Autodesk Inventor part; units mm, degrees
ref_plane "YZ Plane" through (0, 0, 0) normal (1, 0, 0) x (0, 1, 0)
ref_plane "XZ Plane" through (0, 0, 0) normal (0, 1, 0) x (-1, 0, 0)
ref_plane "XY Plane" through (0, 0, 0) normal (0, 0, 1) x (1, 0, 0)
sketch "スケッチ1" plane through (0, 0, 0) normal (0, 0, 1) x (1, 0, 0)
  circle A0 centre (89.1334, 60.2981) radius 8.025
  arc A1 (110.4927, 37.2495) -> (107.5312, 48.5254) centre (107.6371, 42.5263) ccw
  arc A2 (106.5859, 49.1517) -> (107.5312, 48.5254) centre (107.5135, 49.5253) ccw
  line L0 (106.5859, 49.1517) -> (100.2878, 64.7903)
  arc A3 (100.2878, 64.7903) -> (96.6592, 69.6769) centre (89.1334, 60.2981) ccw
  line L1 (96.6592, 69.6769) -> (61.7006, 97.7286)
  arc A4 (61.7006, 97.7286) -> (50.6268, 86.1987) centre (56.6782, 91.4695) ccw
  line L2 (50.6268, 86.1987) -> (79.2604, 53.3248)
  arc A5 (79.3697, 53.1725) -> (79.2604, 53.3248) centre (78.5063, 52.668) ccw
  line L3 (79.3697, 53.1725) -> (86.5144, 40.9457)
  arc A6 (86.5144, 40.9457) -> (87.5386, 39.6454) centre (91.6947, 43.9728) ccw
  line L4 (87.5386, 39.6454) -> (105.5692, 22.328)
  arc A7 (105.5692, 22.328) -> (111.1188, 32.4913) centre (109.7254, 26.6553) ccw
  arc A8 (110.3596, 33.3335) -> (111.1188, 32.4913) centre (111.3511, 33.464) ccw
  line L5 (110.3596, 33.3335) -> (109.9772, 36.2396)
  arc A9 (110.4927, 37.2495) -> (109.9772, 36.2396) centre (110.9687, 36.37) ccw
  circle A10 centre (68.955, 78.0364) radius 1.25
  circle A11 centre (109.7254, 26.6553) radius 3.025
  circle A12 centre (107.6371, 42.5263) radius 3.025
  circle A13 centre (91.6947, 43.9728) radius 3.025
  circle A14 centre (56.6782, 91.4695) radius 1.25
  arc A15 (83.1457, 72.8964) -> (83.5589, 72.581) centre (90.3437, 81.8972) ccw
  arc A16 (83.1457, 72.8964) -> (74.4673, 77.9243) centre (62.1124, 46.5952) ccw
  arc A17 (74.4673, 77.9243) -> (73.1203, 77.1926) centre (74.1004, 76.994) ccw
  arc A18 (68.4822, 73.8128) -> (73.1203, 77.1926) centre (68.955, 78.0364) ccw
  arc A19 (68.4822, 73.8128) -> (67.371, 72.8351) centre (68.3709, 72.819) ccw
  line L6 (67.371, 72.8351) -> (67.3568, 71.9495)
  arc A20 (67.3568, 71.9495) -> (67.6026, 71.2766) centre (68.3567, 71.9334) ccw
  line L7 (67.6026, 71.2766) -> (75.5898, 62.1066)
  arc A21 (75.5898, 62.1066) -> (77.3258, 62.5741) centre (76.3438, 62.7634) ccw
  arc A22 (83.4434, 70.8917) -> (77.3258, 62.5741) centre (89.1334, 60.2981) ccw
  arc A23 (83.4434, 70.8917) -> (83.5589, 72.581) centre (82.9702, 71.7727) ccw
  arc A24 (97.4697, 45.6005) -> (95.5411, 48.5777) centre (91.6947, 43.9728) ccw
  arc A25 (97.4697, 45.6005) -> (98.3419, 44.8759) centre (98.4322, 45.8718) ccw
  line L8 (98.3419, 44.8759) -> (101.261, 44.611)
  arc A26 (101.261, 44.611) -> (102.2493, 45.1668) centre (101.3514, 45.6069) ccw
  arc A27 (103.6511, 47.011) -> (102.2493, 45.1668) centre (107.6371, 42.5263) ccw
  arc A28 (103.6511, 47.011) -> (103.9749, 47.6045) centre (102.9868, 47.7585) ccw
  line L9 (103.9749, 47.6045) -> (101.3375, 54.1532)
  arc A29 (101.3375, 54.1532) -> (99.5442, 54.2801) centre (100.4099, 53.7796) ccw
  arc A30 (95.641, 50.1861) -> (99.5442, 54.2801) centre (89.1334, 60.2981) ccw
  arc A31 (95.641, 50.1861) -> (95.5411, 48.5777) centre (96.1822, 49.3452) ccw
  circle A32 centre (89.1334, 60.2981) radius 8.025
  arc A33 (110.4927, 37.2495) -> (107.5312, 48.5254) centre (107.6371, 42.5263) ccw
  arc A34 (110.4927, 37.2495) -> (109.9772, 36.2396) centre (110.9687, 36.37) ccw
  line L10 (109.9772, 36.2396) -> (110.3596, 33.3335)
  arc A35 (110.3596, 33.3335) -> (111.1188, 32.4913) centre (111.3511, 33.464) ccw
  arc A36 (105.5692, 22.328) -> (111.1188, 32.4913) centre (109.7254, 26.6553) ccw
  line L11 (105.5692, 22.328) -> (87.5386, 39.6454)
  arc A37 (86.5144, 40.9457) -> (87.5386, 39.6454) centre (91.6947, 43.9728) ccw
  line L12 (86.5144, 40.9457) -> (79.3697, 53.1725)
  arc A38 (79.3697, 53.1725) -> (79.2604, 53.3248) centre (78.5063, 52.668) ccw
  line L13 (79.2604, 53.3248) -> (64.3325, 70.4633)
  line L14 (64.3325, 70.4633) -> (64.5025, 81.0256)
  arc A39 (66.7554, 82.9773) -> (64.5025, 81.0256) centre (66.5022, 80.9934) ccw
  arc A40 (85.0194, 75.2394) -> (66.7554, 82.9773) centre (62.1124, 46.5952) ccw
  arc A41 (85.0194, 75.2394) -> (87.9169, 73.7249) centre (90.3437, 81.8972) ccw
  line L15 (87.9169, 73.7249) -> (92.6989, 72.3049)
  arc A42 (93.9266, 71.8696) -> (92.6989, 72.3049) centre (89.1334, 60.2981) ccw
  line L16 (93.9266, 71.8696) -> (96.6592, 69.6769)
  arc A43 (100.2878, 64.7903) -> (96.6592, 69.6769) centre (89.1334, 60.2981) ccw
  line L17 (100.2878, 64.7903) -> (106.5859, 49.1517)
  arc A44 (106.5859, 49.1517) -> (107.5312, 48.5254) centre (107.5135, 49.5253) ccw
  line L18 (107.3853, 32.9421) -> (107.0029, 35.8482)
  arc A45 (107.0029, 35.8482) -> (106.2437, 36.6904) centre (106.0114, 35.7177) ccw
  arc A46 (101.8621, 40.8987) -> (106.2437, 36.6904) centre (107.6371, 42.5263) ccw
  arc A47 (101.8621, 40.8987) -> (100.9899, 41.6233) centre (100.8996, 40.6274) ccw
  line L19 (100.9899, 41.6233) -> (98.0708, 41.8881)
  arc A48 (98.0708, 41.8881) -> (97.0825, 41.3323) centre (97.9804, 40.8922) ccw
  arc A49 (94.6542, 38.7535) -> (97.0825, 41.3323) centre (91.6947, 43.9728) ccw
  arc A50 (94.6542, 38.7535) -> (94.4548, 37.1624) centre (95.1475, 37.8836) ccw
  line L20 (94.4548, 37.1624) -> (102.8092, 29.1384)
  arc A51 (102.8092, 29.1384) -> (104.391, 29.4019) centre (103.5019, 29.8597) ccw
  arc A52 (106.8698, 31.9322) -> (104.391, 29.4019) centre (109.7254, 26.6553) ccw
  arc A53 (106.8698, 31.9322) -> (107.3853, 32.9421) centre (106.3938, 32.8117) ccw
  circle A54 centre (107.6371, 42.5263) radius 3.025
  circle A55 centre (68.955, 78.0364) radius 1.25
  circle A56 centre (91.6947, 43.9728) radius 3.025
  circle A57 centre (109.7254, 26.6553) radius 3.025
  line L21 (61.7006, 97.7286) -> (93.9266, 71.8696)
  arc A58 (93.9266, 71.8696) -> (92.6989, 72.3049) centre (89.1334, 60.2981) ccw
  line L22 (87.9169, 73.7249) -> (92.6989, 72.3049)
  arc A59 (85.0194, 75.2394) -> (87.9169, 73.7249) centre (90.3437, 81.8972) ccw
  arc A60 (85.0194, 75.2394) -> (66.7554, 82.9773) centre (62.1124, 46.5952) ccw
  arc A61 (66.7554, 82.9773) -> (64.5025, 81.0256) centre (66.5022, 80.9934) ccw
  line L23 (64.3325, 70.4633) -> (64.5025, 81.0256)
  line L24 (64.3325, 70.4633) -> (50.6268, 86.1987)
  arc A62 (61.7006, 97.7286) -> (50.6268, 86.1987) centre (56.6782, 91.4695) ccw
  circle A63 centre (56.6782, 91.4695) radius 4
  point P0 (0, 0)
  point P1 (0, 0)
extrude "押し出し1" add sketch "スケッチ1" against normal blind 3 contours A9 L5 A8 A7 L4 A6 L3 A5 L2 L14 A39 A40 A41 L15 A42 L1 A3 L0 A2 A1 | A42 L15 A41 A40 A39 L14 L2 A4 L1 | A15 A23 A22 A21 L7 A20 L6 A19 A18 A17 A16 | A24 A31 A30 A29 L9 A28 A27 A26 L8 A25 | A53 A52 A51 L20 A50 A49 A48 L19 A47 A46 A45 L18 | A63
extrude "押し出し2" cut sketch "スケッチ1" against normal blind 2 contours A42 L15 A41 A40 A39 L14 L2 A4 L1
extrude "押し出し3" cut sketch "スケッチ1" against normal blind 2.5 contours A15 A23 A22 A21 L7 A20 L6 A19 A18 A17 A16 | A24 A31 A30 A29 L9 A28 A27 A26 L8 A25 | A53 A52 A51 L20 A50 A49 A48 L19 A47 A46 A45 L18
hole "穴1" at (68.955, 78.0364, 0) at (56.6782, 91.4695, 0) direction (0, 0, -1) diameter 3 depth 12 tip angle 118
sketch "スケッチ2" plane through (0, 0, -2) normal (0, 0, 1) x (1, 0, 0)
  circle A0 centre (68.955, 78.0364) radius 1.5
  circle A1 centre (56.6782, 91.4695) radius 1.5
  arc A2 (94.6542, 38.7535) -> (94.4548, 37.1624) centre (95.1475, 37.8836) ccw
  line L0 (94.4548, 37.1624) -> (102.8092, 29.1384)
  arc A3 (102.8092, 29.1384) -> (104.391, 29.4019) centre (103.5019, 29.8597) ccw
  arc A4 (106.8698, 31.9322) -> (104.391, 29.4019) centre (109.7254, 26.6553) ccw
  arc A5 (106.8698, 31.9322) -> (107.3853, 32.9421) centre (106.3938, 32.8117) ccw
  line L1 (107.3853, 32.9421) -> (107.0029, 35.8482)
  arc A6 (107.0029, 35.8482) -> (106.2437, 36.6904) centre (106.0114, 35.7177) ccw
  arc A7 (101.8621, 40.8987) -> (106.2437, 36.6904) centre (107.6371, 42.5263) ccw
  arc A8 (101.8621, 40.8987) -> (100.9899, 41.6233) centre (100.8996, 40.6274) ccw
  line L2 (100.9899, 41.6233) -> (98.0708, 41.8881)
  arc A9 (98.0708, 41.8881) -> (97.0825, 41.3323) centre (97.9804, 40.8922) ccw
  arc A10 (94.6542, 38.7535) -> (97.0825, 41.3323) centre (91.6947, 43.9728) ccw
  arc A11 (95.641, 50.1861) -> (95.5411, 48.5777) centre (96.1822, 49.3452) ccw
  arc A12 (97.4697, 45.6005) -> (95.5411, 48.5777) centre (91.6947, 43.9728) ccw
  arc A13 (97.4697, 45.6005) -> (98.3419, 44.8759) centre (98.4322, 45.8718) ccw
  line L3 (98.3419, 44.8759) -> (101.261, 44.611)
  arc A14 (101.261, 44.611) -> (102.2493, 45.1668) centre (101.3514, 45.6069) ccw
  arc A15 (103.6511, 47.011) -> (102.2493, 45.1668) centre (107.6371, 42.5263) ccw
  arc A16 (103.6511, 47.011) -> (103.9749, 47.6045) centre (102.9868, 47.7585) ccw
  line L4 (103.9749, 47.6045) -> (101.3375, 54.1532)
  arc A17 (101.3375, 54.1532) -> (99.5442, 54.2801) centre (100.4099, 53.7796) ccw
  arc A18 (95.641, 50.1861) -> (99.5442, 54.2801) centre (89.1334, 60.2981) ccw
  line L5 (67.371, 72.8351) -> (67.3568, 71.9495)
  arc A19 (67.3568, 71.9495) -> (67.6026, 71.2766) centre (68.3567, 71.9334) ccw
  line L6 (67.6026, 71.2766) -> (75.5898, 62.1066)
  arc A20 (75.5898, 62.1066) -> (77.3258, 62.5741) centre (76.3438, 62.7634) ccw
  arc A21 (83.4434, 70.8917) -> (77.3258, 62.5741) centre (89.1334, 60.2981) ccw
  arc A22 (83.4434, 70.8917) -> (83.5589, 72.581) centre (82.9702, 71.7727) ccw
  arc A23 (83.1457, 72.8964) -> (83.5589, 72.581) centre (90.3437, 81.8972) ccw
  arc A24 (83.1457, 72.8964) -> (74.4673, 77.9243) centre (62.1124, 46.5952) ccw
  arc A25 (74.4673, 77.9243) -> (73.1203, 77.1926) centre (74.1004, 76.994) ccw
  arc A26 (68.4822, 73.8128) -> (73.1203, 77.1926) centre (68.955, 78.0364) ccw
  arc A27 (68.4822, 73.8128) -> (67.371, 72.8351) centre (68.3709, 72.819) ccw
  circle A28 centre (56.6782, 91.4695) radius 4
  line L7 (64.3325, 70.4633) -> (64.5025, 81.0256)
  arc A29 (66.7554, 82.9773) -> (64.5025, 81.0256) centre (66.5022, 80.9934) ccw
  arc A30 (85.0194, 75.2394) -> (66.7554, 82.9773) centre (62.1124, 46.5952) ccw
  arc A31 (85.0194, 75.2394) -> (87.9169, 73.7249) centre (90.3437, 81.8972) ccw
  line L8 (87.9169, 73.7249) -> (92.6989, 72.3049)
  arc A32 (93.9266, 71.8696) -> (92.6989, 72.3049) centre (89.1334, 60.2981) ccw
  line L9 (61.7006, 97.7286) -> (93.9266, 71.8696)
  arc A33 (61.7006, 97.7286) -> (50.6268, 86.1987) centre (56.6782, 91.4695) ccw
  line L10 (64.3325, 70.4633) -> (50.6268, 86.1987)
  line L11 (79.2604, 53.3248) -> (64.3325, 70.4633)
  arc A34 (79.3697, 53.1725) -> (79.2604, 53.3248) centre (78.5063, 52.668) ccw
  line L12 (86.5144, 40.9457) -> (79.3697, 53.1725)
  arc A35 (86.5144, 40.9457) -> (87.5386, 39.6454) centre (91.6947, 43.9728) ccw
  line L13 (105.5692, 22.328) -> (87.5386, 39.6454)
  arc A36 (105.5692, 22.328) -> (111.1188, 32.4913) centre (109.7254, 26.6553) ccw
  arc A37 (110.3596, 33.3335) -> (111.1188, 32.4913) centre (111.3511, 33.464) ccw
  line L14 (109.9772, 36.2396) -> (110.3596, 33.3335)
  arc A38 (110.4927, 37.2495) -> (109.9772, 36.2396) centre (110.9687, 36.37) ccw
  arc A39 (110.4927, 37.2495) -> (107.5312, 48.5254) centre (107.6371, 42.5263) ccw
  arc A40 (106.5859, 49.1517) -> (107.5312, 48.5254) centre (107.5135, 49.5253) ccw
  line L15 (100.2878, 64.7903) -> (106.5859, 49.1517)
  arc A41 (100.2878, 64.7903) -> (96.6592, 69.6769) centre (89.1334, 60.2981) ccw
  line L16 (93.9266, 71.8696) -> (96.6592, 69.6769)
  circle A42 centre (89.1334, 60.2981) radius 8.025
  circle A43 centre (109.7254, 26.6553) radius 3.025
  circle A44 centre (107.6371, 42.5263) radius 3.025
  circle A45 centre (91.6947, 43.9728) radius 3.025
  point P0 (0, 0)
extrude "押し出し4" add sketch "スケッチ2" along normal blind 0.25 contours L10 A33 L9 A32 L8 A31 A30 A29 L7
chamfer "面取り1" distance 1.75 angle 45 2 edges at (68.955, 79.5364, -3) (56.6782, 92.9695, -3)
properties part number "アーム 中間節(ミラー)" material "アルミニウム 7075"
Source: CAD feature listing. Evaluate the final solid. Frame: model axes, mm. A direction names the side the tool comes from. Give positions to 0.01 mm unless a question says otherwise; leave off trailing zeros. Loops run counter-clockwise (first coordinate to the right, second up) from the corner with the lowest first, then second, coordinate; pieces in that order, holes last. Notation, with made-up numbers: (-40, 7.5) - (3, 7.5) arc R26 cw to (3, 36.5) - close; hole circle Ø4 at (-39.75, 38). An arc over 180 degrees is marked (long way). Use CSV: the item, a comma, the result in double quotes. Start each with the question number.
1. Section D-D (y = 31). Output: boundary loops of the cut face in (x, z), then the cut area to 3 significant figures.
2. Section B-B (x = 63). Output: boundary loops of the cut face in (y, z).
3. Reachability of faces 1 (the flat face through (110.17, 34.77, -1.48)), 2 (the cylindrical face through (83.967, 71.69, -1.232)), 3 (the cylindrical face through (86.374, 74.353, -0.863)) from +Z, -Z, +X, -X, +Y, -Y: full face, straight path, thin tool, end or side. Return the list, or none.
4. Section C-C (y = 84). Output: boundary loops of the cut face in (x, z).
5. Ray query, L1, parallel to X at y = 77, z = -0.9; L2, parallel to X at y = 67, z = -0.3; L3, parallel to Y at x = 99, z = -1.2. Return the intervals inside material, ascending.
6. Pin query (flat end, axial travel): pin 1 (4 mm diameter, centred on x = 79.5, y = 81.5, fed in from +Z); pin 2 (4 mm diameter, centred on x = 71.5, y = 71, fed in from +Z); pin 3 (5 mm diameter, centred on x = 68.96, y = 78.04, fed in from -Z). Return the tip coordinate at first contact, or that it passes through.
7. Draft query along Y for faces 4 (the flat face through (56.6, 89.7, 0)), 5 (the cylindrical face through (76.55, 80.31, -0.86)), 6 (the cylindrical face through (100.496, 54.776, -1.232)). Return one class per face: +Y half, -Y half, draft (parallel to the pull), parting line (faces both ways), or undercut.
8. Section A-A (y = 57). Output: boundary loops of the cut face in (x, z).
Response:
1,outline,"(96.54, -3) - (113.86, -3) - (113.86, 0) - (105.59, 0) - (105.59, -2.5) - (100.87, -2.5) - (100.87, 0) - (96.54, 0) - close"
1,area,"40.2 mm²"
2,outline,"(71.99, -3) - (96.69, -3) - (96.69, -1.75) - (71.99, -1.75) - close"
3,face 1,"+Z, -Z, +X"
3,face 2,"+Z"
3,face 3,"+Z, +X, +Y"
4,outline,"(52.54, -3) - (78.81, -3) - (78.81, -1.75) - (52.54, -1.75) - close"
5,L1,"64.44 to 67.87, 70.04 to 73.08, 76.59 to 82.63"
5,L2,"67.35 to 71.33, 79.15 to 84.72, 93.55 to 99.12"
5,L3,"28.64 to 32.8, 41.8 to 44.82, 53.42 to 67.17"
6,pin 1,"z = -1.75"
6,pin 2,"z = -2.5"
6,pin 3,"z = -2.26"
7,face 4,"draft"
7,face 5,"+Y half"
7,face 6,"undercut"
8,outline,"(76.06, -3) - (81.82, -3) - (81.82, 0) - (76.06, 0) - close; (96.45, -3) - (103.43, -3) - (103.43, 0) - (96.45, 0) - close"
